Can you work these out from the model? Positions are in its coordinate system, mm. Coordinates: 2 decimals unless noted, no trailing zeros. Write each loop counter-clockwise with the first axis right and the second up, starting at its lowest first coordinate (ties: lowest second). Pieces come first, ordered by that corner, then holes. Notation, with made-up numbers: (85.5, -27.75) - (126.5, -27.75) arc R11 ccw to (126.5, -12.75) - close; hole circle Ø9 at (62, -29). An arc over 180 degrees is marked (long way). Write each question's results on one line, items separated by ' | '. Start each with the question number.
```python
from build123d import *

# Parameters (mm, degrees)
F0_R            = 114.3
F0_R_2          = 1.7272
F0_R_3          = 12.7
F1_DEPTH        = 3.175
F2_R            = 1.7272
F3_DEPTH        = 3.175
F3_COPIES_COUNT = 8
F5_DEPTH        = 3.175
F5_COPIES_COUNT = 8


# Not quite as in the source:
# - a pattern or mirror of a feature is missing from the dataset's text; its kind, count and spacing are read off the source's solid


with BuildPart() as f1:
    # F0 (on Top) → F1 (new body)
    with BuildSketch(Plane.XY):
        Circle(F0_R)
        with Locations((-12.909118174, -12.909118174)):
            Circle(F0_R_2, mode=Mode.SUBTRACT)
        with Locations((12.909118174, -12.909118174)):
            Circle(F0_R_2, mode=Mode.SUBTRACT)
        with Locations((-12.909118174, 12.909118174)):
            Circle(F0_R_2, mode=Mode.SUBTRACT)
        Circle(F0_R_3, mode=Mode.SUBTRACT)
        with Locations((12.909118174, 12.909118174)):
            Circle(F0_R_2, mode=Mode.SUBTRACT)
    extrude(amount=F1_DEPTH)

    # F2 (on face) → F3 (cut, through all)
    with BuildSketch(Plane.XY.offset(3.175)):
        with Locations((-104.2084193553, 12.676744072)):
            Circle(F2_R)
    f3 = extrude(amount=-F3_DEPTH, mode=Mode.SUBTRACT)

    # F3_copies: F3 ×8 about axis
    f3_copies_axis = Axis((0, 0, 0), (0, 0, 1))
    for i in range(1, F3_COPIES_COUNT):
        add(f3.rotate(f3_copies_axis, i * 360 / F3_COPIES_COUNT), mode=Mode.SUBTRACT)

    # F4 (on face) → F5 (cut, through all)
    with BuildSketch(Plane.XY.offset(3.175)):
        with BuildLine():
            ThreePointArc((-86.3999070415, -67.6589569107), (-87.3583729083, -64.0047703869), (-85.3543905267, -60.8023040588))
            ThreePointArc((-85.3543905267, -60.8023040588), (-82.8464143249, -50.5540157704), (-92.7324291182, -46.8683585731))
            ThreePointArc((-92.7324291182, -46.8683585731), (-94.7342307933, -46.0827839435), (-94.1165439867, -44.0229780172))
            ThreePointArc((-94.1165439867, -44.0229780172), (-90.7433842392, -34.3836080304), (-99.6573570235, -29.3999598059))
            ThreePointArc((-99.6573570235, -29.3999598059), (-101.4849334974, -28.2666894598), (-100.5063583602, -26.3518191911))
            ThreePointArc((-100.5063583602, -26.3518191911), (-95.4522238114, -17.4776215154), (-103.3228234926, -10.9699859169))
            ThreePointArc((-103.3228234926, -10.9699859169), (-104.9164008036, -9.5260853666), (-103.6089432811, -7.8187798076))
            ThreePointArc((-103.6089432811, -7.8187798076), (-97.0517244749, 0.4468259777), (-104.4965013095, 7.922965045))
            ThreePointArc((-104.4965013095, 7.922965045), (-107.8674695554, 9.6283415588), (-108.9360674025, 13.2518529234))
            Line((-108.9360674025, 13.2518529234), (-113.463553135, 13.8026124328))
            ThreePointArc((-113.463553135, 13.8026124328), (-110.1086855289, -30.6686708402), (-89.9907686886, -70.47092699))
            Line((-89.9907686886, -70.47092699), (-86.3999070415, -67.6589569107))
        make_face()
    f5 = extrude(amount=-F5_DEPTH, mode=Mode.SUBTRACT)

    # F5_copies: F5 ×8 about axis
    f5_copies_axis = Axis((0, 0, 0), (0, 0, 1))
    for i in range(1, F5_COPIES_COUNT):
        add(f5.rotate(f5_copies_axis, i * 360 / F5_COPIES_COUNT), mode=Mode.SUBTRACT)


solid = f1.part
```
Q1. If we section it at A-A (x = 0): Please give me the cut outline in (y, z) (3 decimals).
Q2. I'm going to push flat-ended pins straight in: pin 1 Ø10 at (x, y) = (69.5, -79.5) entering from -Z; pin 2 Ø1 at (y, z) = (64, 1.5) entering from +X; pin 3 Ø1.5 at (y, z) = (-4.5, 1.5) entering from -X. Where does each tip first touch, or does it pass through?
Q3. I need wall thicknesses on line 1 along Y through (x, z) = (-26, 2); line 2 along X through (y, z) = (99, 2.1); line 3 along X through (y, z) = (9, 1). Which ranges of each line are inside material? Lowest first, please. Write a range as from..to.
Q4. If we section it at C-C (z = 0.6): Count the separate pieces of the cut face and the enclosed holes in it, then the cut area to 3 significant figures.
Q5. Thinking about a two-plate mould opening in Y: for faces 1 (the face through (23, 2, 0)), 2 (the face through (-0.285, -97.044, 1.61)), 3 (the face through (-95.426, -17.631, 1.61)), which applies, pulls with the +Y half, pulls with the -Y half, needs draft (parallel to the pull), parting line crosses it, or undercut?
Answer list:
1) outline: (-97.039, 0) - (-12.7, 0) - (-12.7, 3.175) - (-97.039, 3.175) - close; (12.7, 0) - (97.039, 0) - (97.039, 3.175) - (12.7, 3.175) - close
2) pin 1: stops at z = 0 | pin 2: stops at x = 87.41 | pin 3: stops at x = -99.02
3) line 1: y = -94.02..99.7 | line 2: x = -29.3..-25.6, -12.21..-5.22, 5.22..17.79, 32.6..35.17 | line 3: x = -107.24..-8.96, 8.96..104.88
4) separate pieces: 1 | enclosed holes: 13 | area: 31,200 mm2
5) face 1: needs draft | face 2: pulls with the -Y half | face 3: undercut
